The model under review builds one solid part; all positions refer to its coordinate system, in mm. Face numbers are marked on the shaded views. A direction names the side the tool comes from. Round coordinates to 2 decimals unless told otherwise and drop trailing zeros. Write each loop counter-clockwise with the first axis right and the second up, starting at its lowest first coordinate (ties: lowest second). Pieces come first, ordered by that corner, then holes.
Item 1: Add section A-A (z = 7.5). Give the boundary of the cut face in (x, y).
Item 2: Draft analysis for pull direction Z (two halves, no side actions). For the marked faces 1, 2 and 3, state which applies: +Z half, -Z half, draft (parallel to the pull), parting line (faces both ways), or undercut.
Item 3: Add section D-D (z = 0). Give the boundary of the cut face in (x, y), plus the area to 3 significant figures.
Item 4: Add section B-B (x = 0). Give the boundary of the cut face in (y, z), plus the area to 3 significant figures.
Item 5: Clearance check with flat-ended pins moving along their axes: pin 1 Ø2 at (x, z) = (12.5, 12.5) entering from +Y; pin 2 Ø3 at (x, y) = (-8, 27) entering from +Z; pin 3 Ø1.5 at (x, z) = (-12.5, 12.5) entering from -Y. State where each tip first meets the part, or that it passes through.
Item 6: To check wall thickness, follow L1, parallel to Z at x = -12.5, y = 3.5; L2, parallel to X at y = 5.25, z = 12.5; L3, parallel to X at y = 5, z = 12. State the ranges of each line that lie inside material, in increasing order.
Item 7: Add section C-C (y = 14). Give the boundary of the cut face in (x, z).
Item 8: Machinability: for the marked faces 4 and 5, which of the approach directions +Z, -Z, +X, -X, +Y, -Y give a long, thin tool a straight path to every point of the face, cutting with its end or side? Answer none if there is none.
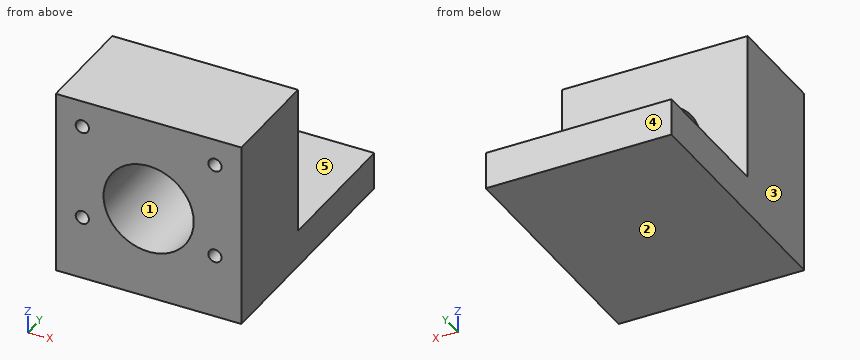
```python
from build123d import *

# Parameters (mm, degrees)
SKETCH1_W             = 35
SKETCH1_H             = 35
BOSS_EXTRUDE1_DEPTH   = 20
SKETCH2_W             = 35
SKETCH2_H             = 7
BOSS_EXTRUDE2_DEPTH   = 27
SKETCH3_R             = 8.5
CUT_EXTRUDE1_DEPTH    = 20
M3_TAPPED_HOLE1_D     = 2.5
M3_TAPPED_HOLE1_DEPTH = 7.5
M3_TAPPED_HOLE1_TIP   = 0.751075774


with BuildPart() as part:
    # Sketch1 → Boss-Extrude1 (new body)
    with BuildSketch(Plane(origin=(0, 0, 0), x_dir=(1, 0, 0), z_dir=(0, 1, 0))):
        Rectangle(SKETCH1_W, SKETCH1_H)
    extrude(amount=BOSS_EXTRUDE1_DEPTH)

    # Sketch2 → Boss-Extrude2 (add)
    with BuildSketch(Plane(origin=(0, 20, 0), x_dir=(1, 0, 0), z_dir=(0, 1, 0))):
        with Locations((0, 14)):
            Rectangle(SKETCH2_W, SKETCH2_H)
    extrude(amount=BOSS_EXTRUDE2_DEPTH)

    # Sketch3 → Cut-Extrude1 (cut)
    with BuildSketch(Plane.XZ):
        Circle(SKETCH3_R)
    extrude(amount=-CUT_EXTRUDE1_DEPTH, mode=Mode.SUBTRACT)

    # M3 Tapped Hole1
    with Locations(Plane(origin=(0, 0, 0), x_dir=(-1, 0, 0), z_dir=(0, -1, 0))):
        with Locations((-12.5, 5.5), (12.5, 5.5), (12.5, -12.5), (-12.5, -12.5)):
            Hole(M3_TAPPED_HOLE1_D / 2, depth=M3_TAPPED_HOLE1_DEPTH)
            with Locations((0, 0, -(M3_TAPPED_HOLE1_DEPTH + M3_TAPPED_HOLE1_TIP / 2))):  # 118° drill point
                Cone(0, M3_TAPPED_HOLE1_D / 2, M3_TAPPED_HOLE1_TIP, mode=Mode.SUBTRACT)


solid = part.part
```
Numbers:
1. outline: (-17.5, 0) - (-4, 0) - (-4, 20) - (-17.5, 20) - close; (4, 0) - (17.5, 0) - (17.5, 20) - (4, 20) - close
2. face 1: undercut
2. face 2: -Z half
2. face 3: draft
3. outline: (-17.5, 0) - (-8.5, 0) - (-8.5, 20) - (-17.5, 20) - close; (8.5, 0) - (17.5, 0) - (17.5, 20) - (8.5, 20) - close
3. area: 360 mm2
4. outline: (0, -17.5) - (47, -17.5) - (47, -10.5) - (20, -10.5) - (20, -8.5) - (0, -8.5) - close; (0, 8.5) - (20, 8.5) - (20, 17.5) - (0, 17.5) - close
4. area: 549 mm2
5. pin 1: stops at y = 20
5. pin 2: stops at z = -10.5
5. pin 3: stops at y = 7.8
6. L1: z = -17.5 to -6.75, -4.25 to 11.25, 13.75 to 17.5
6. L2: x = -17.5 to -13.75, -11.25 to 11.25, 13.75 to 17.5
6. L3: x = -17.5 to -13.65, -11.35 to 11.35, 13.65 to 17.5
7. outline: (-17.5, -17.5) - (17.5, -17.5) - (17.5, 17.5) - (-17.5, 17.5) - close; hole circle Ø17 at (0, 0)
8. face 4: +Z, -Z, +X, -X, +Y
8. face 5: +Z, +X, -X, +Y
